```python
from build123d import *

# Parameters (mm, degrees)
SKETCH1_W           = 42
SKETCH1_H           = 42
BOSS_EXTRUDE1_DEPTH = 40
SKETCH4_R           = 2
CUT_EXTRUDE1_DEPTH  = 4.5
SKETCH2_R           = 11
BOSS_EXTRUDE2_DEPTH = 2
SKETCH3_R           = 2.5
BOSS_EXTRUDE3_DEPTH = 22


with BuildPart() as part:
    # Sketch1 → Boss-Extrude1 (new body)
    with BuildSketch(Plane(origin=(0, 0, 0), x_dir=(1, 0, 0), z_dir=(0, 1, 0))):
        Rectangle(SKETCH1_W, SKETCH1_H)
    extrude(amount=BOSS_EXTRUDE1_DEPTH)

    # Sketch4 → Cut-Extrude1 (cut)
    with BuildSketch(Plane(origin=(0, 40, 0), x_dir=(1, 0, 0), z_dir=(0, 1, 0))):
        with Locations(Location((-15.5, 15.5, 0), (0, 0, 270))):
            Circle(SKETCH4_R)
        with Locations(Location((15.5, 15.5, 0), (0, 0, 270))):
            Circle(SKETCH4_R)
        with Locations(Location((-15.5, -15.5, 0), (0, 0, 270))):
            Circle(SKETCH4_R)
        with Locations(Location((15.5, -15.5, 0), (0, 0, 270))):
            Circle(SKETCH4_R)
    extrude(amount=-CUT_EXTRUDE1_DEPTH, mode=Mode.SUBTRACT)

    # Sketch2 → Boss-Extrude2 (add)
    with BuildSketch(Plane(origin=(0, 40, 0), x_dir=(1, 0, 0), z_dir=(0, 1, 0))):
        with Locations(Location((0, 0, 0), (0, 0, 90))):
            Circle(SKETCH2_R)
    extrude(amount=BOSS_EXTRUDE2_DEPTH)

    # Sketch3 → Boss-Extrude3 (add)
    with BuildSketch(Plane(origin=(0, 42, 0), x_dir=(1, 0, 0), z_dir=(0, 1, 0))):
        with Locations(Location((0, 0, 0), (0, 0, 270))):
            Circle(SKETCH3_R)
    extrude(amount=BOSS_EXTRUDE3_DEPTH)


solid = part.part
```
The listing builds one solid part. Answer for the finished solid, in the listing's coordinates (mm). A direction names the side the tool comes from. Give positions to 0.01 mm unless a question says otherwise; leave off trailing zeros. Order: outer loops, then holes, each group sorted by start corner. A loop starts at its lowest first (then second) coordinate and runs counter-clockwise, first axis right, second up.
1) For faces 5 (the face through (17.483, 37.782, -15.76)), 6 (the face through (0, 64, 0)), determine the directions among +Z, -Z, +X, -X, +Y, -Y from which every point of the face is accessible in a straight line to the end or side of a thin tool.
Reported:
face 5: +Y
face 6: +Z, -Z, +X, -X, +Y
2) Consider line 1 along X through (y, z) = (37.45, -15.5); line 2 along Z through (x, y) = (15, 38). Determine where each line is inside the solid, lowest interval first.
Reported:
line 1: x = -21 to -17.5, -13.5 to 13.5, 17.5 to 21
line 2: z = -21 to -17.44, -13.56 to 13.56, 17.44 to 21
3) Find section C-C on x = 0. Write down the section's boundary in (y, z), then the cut area to 3 significant figures.
Reported:
outline: (0, -21) - (40, -21) - (40, -11) - (42, -11) - (42, -2.5) - (64, -2.5) - (64, 2.5) - (42, 2.5) - (42, 11) - (40, 11) - (40, 21) - (0, 21) - close
area: 1,830 mm2
4) Find section B-B on y = 38.5. Write down the section's boundary in (x, z).
Reported:
outline: (-21, -21) - (21, -21) - (21, 21) - (-21, 21) - close; hole circle Ø4 at (-15.5, -15.5); hole circle Ø4 at (-15.5, 15.5); hole circle Ø4 at (15.5, -15.5); hole circle Ø4 at (15.5, 15.5)
5) Find section D-D on y = 52.5. Write down the section's boundary in (x, z), then the cut area to 3 significant figures.
Reported:
outline: circle Ø5 at (0, 0)
area: 19.6 mm2
6) Determine the mould class of faces 1 (the face through (9, 40, 9)), 2 (the face through (-13.517, 37.782, 15.24)), 3 (the face through (17.483, 37.782, 15.24)), 4 (the face through (0, 20, 21)) for opening direction Z: pulls with the +Z half, pulls with the -Z half, needs draft (parallel to the pull), parting line crosses it, or undercut.
Reported:
face 1: needs draft
face 2: undercut
face 3: undercut
face 4: pulls with the +Z half
7) Given P1, Ø6.5, axis at x = 15.5, z = -15.5, coming from the +Y side; P2, Ø1.2, axis at x = 15.5, z = -16, coming from the +Y side; P3, Ø1.5, axis at x = -4, y = 42, coming from the -Z side, each flat-ended and moving along its own axis, determine where each tip first touches the part or whether it passes through.
Reported:
P1: stops at y = 40
P2: stops at y = 35.5
P3: stops at z = -10.51
8) Find section A-A on z = 0. Write down the section's boundary in (x, y), then the cut area to 3 significant figures.
Reported:
outline: (-21, 0) - (21, 0) - (21, 40) - (11, 40) - (11, 42) - (2.5, 42) - (2.5, 64) - (-2.5, 64) - (-2.5, 42) - (-11, 42) - (-11, 40) - (-21, 40) - close
area: 1,830 mm2
